Geometry check sheet. Reference: the model listing, model coordinates, mm. Face numbers are marked on the shaded views. A direction names the side the tool comes from. Round coordinates to 2 decimals unless told otherwise and drop trailing zeros. Write each loop counter-clockwise with the first axis right and the second up, starting at its lowest first coordinate (ties: lowest second). Pieces come first, ordered by that corner, then holes. Notation, with made-up numbers: (-28, 76.25) -> (-7, 76.25) arc R18 cw to (-7, 101.25) -> close; hole circle Ø4 at (87, 45.25). An arc over 180 degrees is marked (long way). Use a Markdown table: item, result.
```python
from build123d import *

# Parameters (mm, degrees)
SKETCH_R        = 1.75
PAD_DEPTH       = 2
PAD001_DEPTH    = 5
SKETCH002_W     = 61
SKETCH002_H     = 81
PAD002_DEPTH    = 2
PAD003_DEPTH    = 49.3
PAD004_DEPTH    = 2
SKETCH005_W     = 5
SKETCH005_H     = 10
PAD005_DEPTH    = 2
SKETCH006_W     = 51
SKETCH006_H     = 43.3
POCKET_DEPTH    = 81
SKETCH007_W     = 71
SKETCH007_H     = 43.3
POCKET001_DEPTH = 2


with BuildPart() as part:
    # Sketch → Pad (new body)
    with BuildSketch(Plane.XY):
        Polygon((-13.279056, 21), (-13.279056, -21), (-11.547005, -22), (24.826062, -1), (24.826062, 1), (-11.547005, 22), align=None)
        with Locations((-7.279056, 0)):
            Circle(SKETCH_R, mode=Mode.SUBTRACT)
        with Locations((3.639528, 6.303848)):
            Circle(SKETCH_R, mode=Mode.SUBTRACT)
        with Locations((3.639528, -6.303848)):
            Circle(SKETCH_R, mode=Mode.SUBTRACT)
        Polygon((6.558112, 0), (-3.279056, 5.679492), (-3.279056, -5.679492), align=None, mode=Mode.SUBTRACT)
    extrude(amount=PAD_DEPTH)

    # Sketch001 (on Face14 of Pad) → Pad001 (join)
    with BuildSketch(Plane.XY.offset(2)):
        Polygon((-13.279056, 21), (-11.547005, 22), (24.826062, 1), (24.826062, -1), (-11.547005, -22), (-13.279056, -21), align=None)
        Polygon((22.558112, 0), (-11.279056, 19.535898), (-11.279056, -19.535898), align=None, mode=Mode.SUBTRACT)
    extrude(amount=PAD001_DEPTH)

    # Sketch002 (on Face17 of Pad001) → Pad002 (join)
    with BuildSketch(Plane.XY.offset(7)):
        with Locations((-3.5, 0)):
            Rectangle(SKETCH002_W, SKETCH002_H)
        Polygon((-11.279056, 19.535898), (22.558112, 0), (-11.279056, -19.535898), align=None, mode=Mode.SUBTRACT)
    extrude(amount=PAD002_DEPTH)

    # Sketch003 (on Face29 of Pad002) → Pad003 (join)
    with BuildSketch(Plane.XY.offset(9)):
        Polygon((-34, 40.5), (27, 40.5), (27, -40.5), (-34, -40.5), (-34, -38.5), (25, -38.5), (25, 38.5), (-34, 38.5), align=None)
    extrude(amount=PAD003_DEPTH)

    # Sketch004 (on Face38 of Pad003) → Pad004 (join)
    with BuildSketch(Plane.XY.offset(58.3)):
        Polygon((-34, 40.5), (27, 40.5), (27, -40.5), (-34, -40.5), (-34, -35.5), (22, -35.5), (22, 35.5), (-34, 35.5), align=None)
    extrude(amount=PAD004_DEPTH)

    # Sketch005 (on Face30 of Pad004) → Pad005 (join)
    with BuildSketch(Plane(origin=(-34, 0, 0), x_dir=(0, -1, 0), z_dir=(-1, 0, 0))):
        with Locations((-38, 55.3)):
            Rectangle(SKETCH005_W, SKETCH005_H)
        with Locations((38, 55.3)):
            Rectangle(SKETCH005_W, SKETCH005_H)
    extrude(amount=-PAD005_DEPTH)

    # Sketch006 → Pocket (cut)
    with BuildSketch(Plane.XZ.offset(40.5)):
        with Locations((-3.5, 33.65)):
            Rectangle(SKETCH006_W, SKETCH006_H)
    extrude(amount=-POCKET_DEPTH, mode=Mode.SUBTRACT)

    # Sketch007 → Pocket001 (cut)
    with BuildSketch(Plane.YZ.offset(27)):
        with Locations((0, 33.65)):
            Rectangle(SKETCH007_W, SKETCH007_H)
    extrude(amount=-POCKET001_DEPTH, mode=Mode.SUBTRACT)


solid = part.part
```
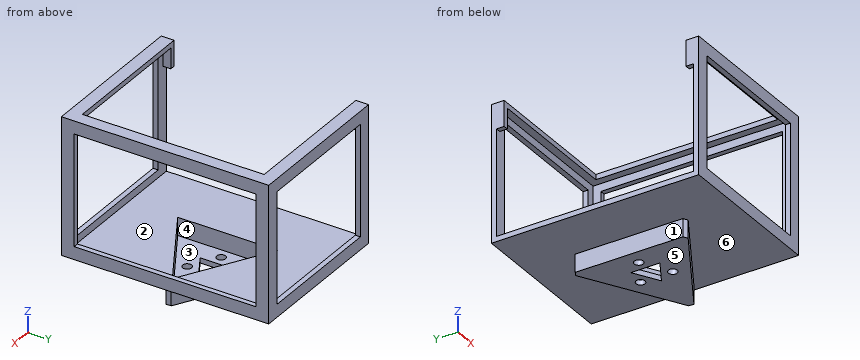
(1) Section check D-D on y = -14. Record the cut outline in (x, z).
A:
| item | result |
|---|---|
| outline | (-34, 7) -> (-13.28, 7) -> (-13.28, 0) -> (2.31, 0) -> (2.31, 7) -> (27, 7) -> (27, 12) -> (25, 12) -> (25, 9) -> (-1.69, 9) -> (-1.69, 2) -> (-11.28, 2) -> (-11.28, 9) -> (-34, 9) -> close; (22, 58.3) -> (25, 58.3) -> (25, 55.3) -> (27, 55.3) -> (27, 60.3) -> (22, 60.3) -> close |
(2) Thickness scan on line 1 (Y direction, x = -7.5, z = 57); line 2 (Z direction, x = 10.5, y = 36); line 3 (X direction, y = 35, z = 10). Record the ranges inside material, lowest first.
A:
| item | result |
|---|---|
| line 1 | y = -40.5 to -38.5, 38.5 to 40.5 |
| line 2 | z = 7 to 9, 58.3 to 60.3 |
| line 3 | x = 25 to 27 |
(3) Section check A-A on y = 23.5. Record the cut outline in (x, z).
A:
| item | result |
|---|---|
| outline | (-34, 7) -> (27, 7) -> (27, 12) -> (25, 12) -> (25, 9) -> (-34, 9) -> close; (22, 58.3) -> (25, 58.3) -> (25, 55.3) -> (27, 55.3) -> (27, 60.3) -> (22, 60.3) -> close |
(4) Section check B-B on x = -26.5. Record the cut outline in (y, z), plus the area to 3 significant figures.
A:
| item | result |
|---|---|
| outline | (-40.5, 7) -> (40.5, 7) -> (40.5, 12) -> (38.5, 12) -> (38.5, 9) -> (-38.5, 9) -> (-38.5, 12) -> (-40.5, 12) -> close; (-40.5, 55.3) -> (-38.5, 55.3) -> (-38.5, 58.3) -> (-35.5, 58.3) -> (-35.5, 60.3) -> (-40.5, 60.3) -> close; (35.5, 58.3) -> (38.5, 58.3) -> (38.5, 55.3) -> (40.5, 55.3) -> (40.5, 60.3) -> (35.5, 60.3) -> close |
| area | 206 mm2 |
(5) Release check for a two-part mould opening along X. For the marked faces 1, 2 and 3 record: +X half, -X half, draft (parallel to the pull), parting line (faces both ways), or undercut.
A:
| item | result |
|---|---|
| face 1 | -X half |
| face 2 | draft |
| face 3 | undercut |
(6) Access from +Z, -Z, +X, -X, +Y, -Y to the whole of each face (thin tool, end or side, straight path). Record for the marked faces 4, 5 and 6.
A:
| item | result |
|---|---|
| face 4 | +Z |
| face 5 | -Z, +X, -X, +Y, -Y |
| face 6 | -Z |
(7) Gauge pin test, flat ends, axial feed: pin 1 Ø1 at (y, z) = (-24, 12) entering from -X; pin 2 Ø3 at (x, y) = (17.5, 9.5) entering from -Z; pin 3 Ø1 at (x, y) = (-24.5, 19) entering from +Z. Record the tip position at first contact, or that the pin passes through.
A:
| item | result |
|---|---|
| pin 1 | stops at x = 25 |
| pin 2 | stops at z = 7 |
| pin 3 | stops at z = 9 |
(8) Section check C-C on x = -6.5. State how many separate pieces and enclosed holes the cut face has, plus the area to 3 significant figures.
A:
| item | result |
|---|---|
| separate pieces | 4 |
| enclosed holes | 0 |
| area | 232 mm2 |
